Geometry: see drawing. Coordinates: mm, zero at the bounding-box minimum. Coordinates: 2 decimals unless noted, no trailing zeros. Order: outer loops, then holes, each group sorted by start corner. A loop starts at its lowest first (then second) coordinate and runs counter-clockwise, first axis right, second up.
Item 1: Ray query, line 1 (Y direction, x = 87.5, z = 1.5); line 2 (Y direction, x = 57.5, z = 1.1); line 3 (Z direction, x = 25, y = 20). Return the intervals inside material, ascending.
Item 2: Section D-D on z = 7.5. Return the cut outline in (x, y), then the cut area to 3 significant figures.
Item 3: Section B-B on y = 9. Return the cut outline in (x, z).
Item 4: Section C-C on x = 57.5. Return the cut outline in (y, z), then the cut area to 4 significant figures.
Item 5: Contact query for flat-ended pins moving along their axis: P1, Ø25, axis at x = 44, y = 37.5, coming from the +Z side; P2, Ø4, axis at y = 19.5, z = 2.5, coming from the +X side; P3, Ø1.5, axis at y = 17, z = 2, coming from the +X side. Output: stop coordinate, or through.
Item 6: Section A-A on x = 77.5. Return the cut outline in (y, z).
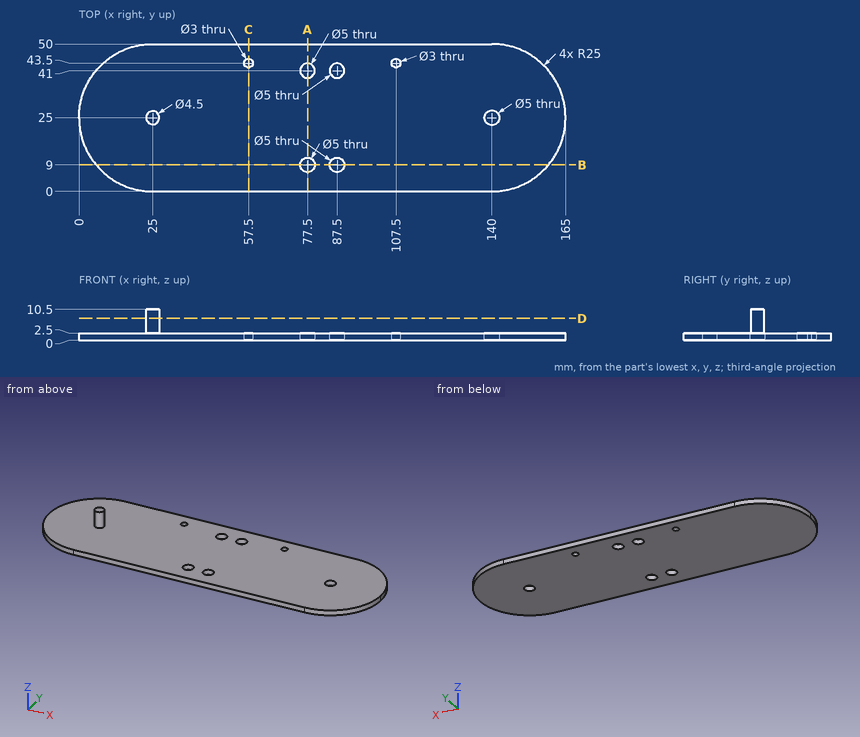
Answer list:
1. line 1: y = 0 to 6.5, 11.5 to 38.5, 43.5 to 50
1. line 2: y = 0 to 42, 45 to 50
1. line 3: z = 0 to 2.5
2. outline: circle Ø4.5 at (25, 25)
2. area: 15.9 mm2
3. outline: (5.79, 0) - (75, 0) - (75, 2.5) - (5.79, 2.5) - close; (80, 0) - (85, 0) - (85, 2.5) - (80, 2.5) - close; (90, 0) - (159.21, 0) - (159.21, 2.5) - (90, 2.5) - close
4. outline: (0, 0) - (42, 0) - (42, 2.5) - (0, 2.5) - close; (45, 0) - (50, 0) - (50, 2.5) - (45, 2.5) - close
4. area: 117.5 mm2
5. P1: stops at z = 2.5
5. P2: stops at x = 164.75
5. P3: stops at x = 163.93
6. outline: (0, 0) - (6.5, 0) - (6.5, 2.5) - (0, 2.5) - close; (11.5, 0) - (38.5, 0) - (38.5, 2.5) - (11.5, 2.5) - close; (43.5, 0) - (50, 0) - (50, 2.5) - (43.5, 2.5) - close
